Source: three-view drawing plus pictorial views. Frame: mm from the lowest corner of the part. Give positions to 0.01 mm unless a question says otherwise; leave off trailing zeros. Write each loop counter-clockwise with the first axis right and the second up, starting at its lowest first coordinate (ties: lowest second). Pieces come first, ordered by that corner, then holes. Notation, with made-up numbers: (24, 24) -> (48, 24) arc R27 ccw to (48, 50) -> close; hole circle Ø7 at (48.5, -11). An arc over 180 degrees is marked (long way). Use a Markdown table: item, result. Add a question column.
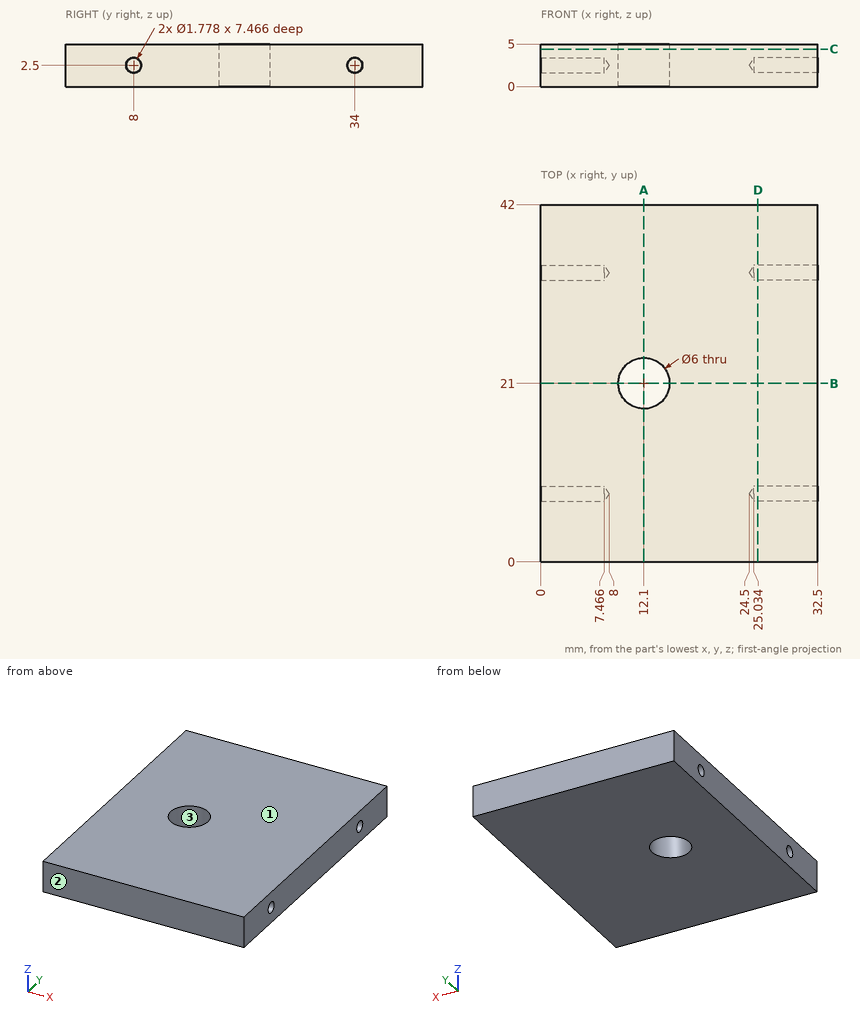
(1) Cut plane C-C on z = 4.4. Return the cut outline in (x, y).
(2) First-contact query: pin 1 Ø7 at (x, y) = (12.1, 21) entering from -Z; pin 2 Ø1.6 at (y, z) = (34, 2.5) entering from -X; pin 3 Ø1.6 at (y, z) = (34, 2.5) entering from +X. Flat tips, straight axial feed; report the tip coordinate or a pass-through.
(3) Mould query, pull axis Y, two halves, no side actions, for the marked faces 1, 2 and 3. Classes: +Y half, -Y half, draft (parallel to the pull), parting line (faces both ways), or undercut.
(4) Cut plane B-B on y = 21. Return the cut outline in (x, z), then the cut area to 4 significant figures.
(5) Material intervals for L1, parallel to Y at x = 27, z = 2.5; L2, parallel to Z at x = 27.25, y = 34; L3, parallel to Y at x = 28.5, z = 3.3, sorted ascending.
(6) Cut plane A-A on x = 12.1. Return the cut outline in (y, z), then the cut area to 3 significant figures.
(7) Cut plane D-D on x = 25.5. Return the cut outline in (y, z), then the cut area to 3 significant figures.
Output:
| question | item | result |
|---|---|---|
| 1 | outline | (0, 0) -> (32.5, 0) -> (32.5, 42) -> (0, 42) -> close; hole circle Ø6 at (12.1, 21) |
| 2 | pin 1 | z = 0 |
| 2 | pin 2 | x = 7.52 |
| 2 | pin 3 | x = 24.98 |
| 3 | face 1 | draft |
| 3 | face 2 | -Y half |
| 3 | face 3 | undercut |
| 4 | outline | (0, 0) -> (9.1, 0) -> (9.1, 5) -> (0, 5) -> close; (15.1, 0) -> (32.5, 0) -> (32.5, 5) -> (15.1, 5) -> close |
| 4 | area | 132.5 mm^2 |
| 5 | L1 | 0 to 7.11, 8.89 to 33.11, 34.89 to 42 |
| 5 | L2 | 0 to 1.61, 3.39 to 5 |
| 5 | L3 | 0 to 7.61, 8.39 to 33.61, 34.39 to 42 |
| 6 | outline | (0, 0) -> (18, 0) -> (18, 5) -> (0, 5) -> close; (24, 0) -> (42, 0) -> (42, 5) -> (24, 5) -> close |
| 6 | area | 180 mm^2 |
| 7 | outline | (0, 0) -> (42, 0) -> (42, 5) -> (0, 5) -> close; hole circle Ø1.78 at (8, 2.5); hole circle Ø1.78 at (34, 2.5) |
| 7 | area | 205 mm^2 |
